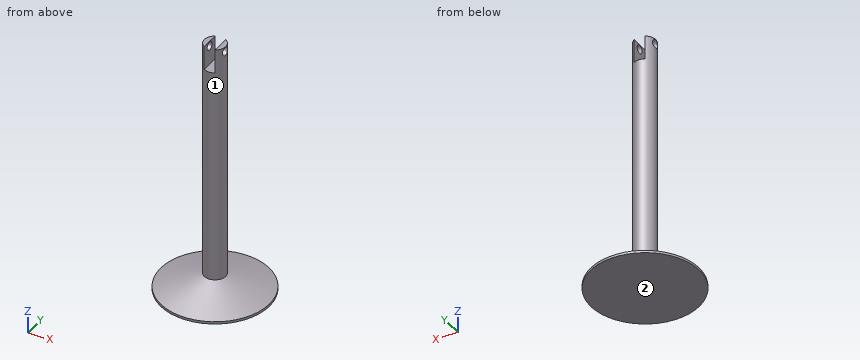
from build123d import *

# Parameters (mm, degrees)
F0_R     = 16.129
F1_DEPTH = 76.2
F4_W     = 3.175
F4_H     = 10.16
F5_DEPTH = 12.7
F6_R     = 1.27
F7_DEPTH = 12.7
F8_DEPTH = 2.54


with BuildPart() as f1:
    # F0 (on Top) → F1 (new body)
    with BuildSketch(Plane.XY):
        Circle(F0_R)
    extrude(amount=F1_DEPTH)

    # F2 (on Front) → F3 (revolve, cut)
    with BuildSketch(Plane.XZ):
        Polygon((-18.3443464339, 0), (-3.175, 4.7896225005), (-3.175, 89.8051410913), (-18.3443464339, 89.8051410913), align=None)
    revolve(axis=Axis((0, 0, 76.2), (0, 0, 1)), mode=Mode.SUBTRACT)

    # F4 (on Front) → F5 (cut, symmetric)
    with BuildSketch(Plane.XZ):
        with Locations((0, 76.7151042819)):
            Rectangle(F4_W, F4_H)
    extrude(amount=F5_DEPTH, both=True, mode=Mode.SUBTRACT)

    # F6 (on Right) → F7 (cut, symmetric)
    with BuildSketch(Plane.YZ):
        with Locations((0, 74.7672840953)):
            Circle(F6_R)
    extrude(amount=F7_DEPTH, both=True, mode=Mode.SUBTRACT)

    # F8 (cut): a face of the model
    f8_faces = [f1.faces().sort_by_distance(p)[0] for p in [
        (0, 0, 71.6351042819),
    ]]
    extrude(f8_faces, amount=-F8_DEPTH, mode=Mode.SUBTRACT)


solid = f1.part
For this review, take the finished solid that the model builds, in its own axes (mm). Face numbers are marked on the shaded views. A direction names the side the tool comes from. Give positions to 0.01 mm unless a question says otherwise; leave off trailing zeros. Order: outer loops, then holes, each group sorted by start corner. A loop starts at its lowest first (then second) coordinate and runs counter-clockwise, first axis right, second up. Notation, with made-up numbers: M 18,33.5 L 34,33.5 A19 ccw 34,54.5 Z; hole C 67,62 d11. An arc over 180 degrees is marked long. Answer in a Markdown table with one row per item. Add a question column.
(1) Consider section C-C on z = 65. State the section outline as (x, y) points (3 decimals), and give its area (3 significant figures).
(2) For pin 1 (3 mm diameter, centred on x = 3.5, z = 41.5, fed in from -Y); pin 2 (1 mm diameter, centred on x = 5, z = 58.5, fed in from +Y); pin 3 (6 mm diameter, centred on y = 0.5, z = 71.5, fed in from +X) (3 decimals); pin 4 (1.6 mm diameter, centred on y = 1.5, z = 73.5, fed in from -X), all flat-tipped, find the tip position at first contact; note any pin that passes through.
(3) Consider section B-B on x = 0. State the section outline as (y, z) points (3 decimals), and give its area (3 significant figures).
(4) Consider section A-A on y = 0. Give the number of separate pieces and of enclosed holes in the cut face, and give its area (3 significant figures).
(5) For the marked faces 1 and 2, list the 3-axis set-ups (+Z, -Z, +X, -X, +Y, -Y) from which the entire face can be reached by the end or side of a thin tool; tool diameter is ignored.
(6) Wall thickness on probe 1 along Z at (x, y) = (-2.8, 0); probe 2 along Y at (x, z) = (0, 24) (3 decimals); probe 3 along Z at (x, y) = (-0.5, 3): over which ranges is each line inside the solid? List them lowest first. Write a range as [from, to].
Evaluation:
| question | item | result |
|---|---|---|
| 1 | outline | C 0,0 d6.35 |
| 1 | area | 31.7 mm^2 |
| 2 | pin 1 | stops at y = -2.47 |
| 2 | pin 2 | passes through |
| 2 | pin 3 | stops at x = 3.175 |
| 2 | pin 4 | stops at x = -3.1 |
| 3 | outline | M -16.129,0 L 16.129,0 L 16.129,0.699 L 3.175,4.79 L 3.175,69.095 L -3.175,69.095 L -3.175,4.79 L -16.129,0.699 Z |
| 3 | area | 510 mm^2 |
| 4 | separate pieces | 3 |
| 4 | enclosed holes | 0 |
| 4 | area | 524 mm^2 |
| 5 | face 1 | +Z |
| 5 | face 2 | -Z, +X, -X, +Y, -Y |
| 6 | probe 1 | z = [0, 73.5], [76.04, 76.2] |
| 6 | probe 2 | y = [-3.175, 3.175] |
| 6 | probe 3 | z = [0, 69.1] |
